Read the model definition and answer for the solid it produces. Units are mm, in the model's axes. A direction names the side the tool comes from. Coordinates: 2 decimals unless noted, no trailing zeros. Loops run counter-clockwise (first coordinate to the right, second up) from the corner with the lowest first, then second, coordinate; pieces in that order, holes last. Notation, with made-up numbers: (41.5, 18) - (80.5, 18) arc R10 cw to (80.5, 34) - close; hole circle Ø11 at (-35, 87.25). An arc over 180 degrees is marked (long way). Use CSV: the item, a comma, the result in double quotes.
Autodesk Inventor part; units mm, degrees
ref_plane "YZ Plane" through (0, 0, 0) normal (1, 0, 0) x (0, 1, 0)
ref_plane "XZ Plane" through (0, 0, 0) normal (0, 1, 0) x (-1, 0, 0)
ref_plane "XY Plane" through (0, 0, 0) normal (0, 0, 1) x (1, 0, 0)
sketch "Эскиз1" plane through (0, 0, 0) normal (0, 1, 0) x (-1, 0, 0)
  line L0 (0, 0) -> (-16, 0)
  line L1 (-16, 0) -> (-16, -7)
  line L2 (-16, -7) -> (0, -7)
  line L3 (0, -7) -> (0, 0)
  circle A0 centre (-13.5, -3.5) radius 1.5
  dimension "d0" = 16
  dimension "d1" = 7
  dimension "d2" = 3
  dimension "d3" = 2.5
  dimension "d4" = 3.5
extrude "Выдавливание1" add sketch "Эскиз1" along normal blind 5
sketch "Эскиз2" plane through (0, 0, 0) normal (0, 1, 0) x (-1, 0, 0)
  line L0 (-16, 0) -> (-16, -7) construction
  line L1 (-16, -7) -> (0, -7) construction
  line L2 (0, -7) -> (0, 0)
  line L3 (0, 0) -> (-16, 0) construction
  circle A0 centre (-13.5, -3.5) radius 1.5 construction
  line L4 (0, 0) -> (-7, 0)
  line L5 (-7, 0) -> (-7, -7)
  line L6 (-7, -7) -> (0, -7)
  line L7 (0, -7) -> (0, 0)
  point P0 (0, -7)
  dimension "d7" = 7
  dimension "d8" = 7
extrude "Выдавливание2" add sketch "Эскиз2" along normal blind 8
sketch "Эскиз3" plane through (0, 0, 0) normal (0, 0, 1) x (1, 0, 0)
  line L0 (0, 0) -> (16, 0) construction
  line L1 (16, 0) -> (16, 5) construction
  line L2 (7, 5) -> (16, 5) construction
  line L3 (7, 5) -> (7, 8) construction
  line L4 (0, 8) -> (7, 8) construction
  line L5 (0, 0) -> (0, 8) construction
  circle A0 centre (3.5, 4.5) radius 1.5
  dimension "d11" = 3
  dimension "d12" = 3.5
  dimension "d13" = 3.5
extrude "Выдавливание3" cut sketch "Эскиз3" against normal blind 7
properties part number "angle_01"
Q1. Find the intervals of material crossed by probe 1 along Z at (x, y) = (13.5, 1.8); probe 2 along X at (y, z) = (3.5, -3.75); probe 3 along Y at (x, z) = (3.5, -5.5), in increasing order. Write a range as [from, to].
Reported:
probe 1,"z = [-7, -5], [-2, 0]"
probe 2,"x = [0, 2.38], [4.62, 12.02], [14.98, 16]"
probe 3,"y = [0, 3], [6, 8]"
Q2. The part is cut by section A-A on z = -3.5. Determine the outline of the cut face in (x, y).
Reported:
outline,"(0, 0) - (12, 0) - (12, 5) - (7, 5) - (7, 8) - (0, 8) - close; (15, 0) - (16, 0) - (16, 5) - (15, 5) - close; hole circle Ø3 at (3.5, 4.5)"
Q3. The part is cut by section D-D on y = 1.75. Determine the outline of the cut face in (x, z), and give its area (3 significant figures).
Reported:
outline,"(0, -7) - (16, -7) - (16, 0) - (0, 0) - close; hole circle Ø3 at (13.5, -3.5)"
area,"105 mm²"
Q4. A tool of negligible diameter and unlimited length cuts with its end or side. For faces 1 (the face through (8, 0, -3)), 2 (the face through (11.6, 5, -3.5)), from which of +Z, -Z, +X, -X, +Y, -Y can it reach the whole face along a straight path? Write none if from no direction.
Reported:
face 1,"+Z, -Z, +X, -X, -Y"
face 2,"+Z, -Z, +X, +Y"
Q5. For a pull along Z with two mould halves and no side action, classify faces 3 (the face through (15, 2.46, -3.57)), 4 (the face through (8, 3, 0)), 5 (the face through (8, 3, -7)), 6 (the face through (16, 2, -3)) as +Z half, -Z half, draft (parallel to the pull), parting line (faces both ways), or undercut.
Reported:
face 3,"undercut"
face 4,"+Z half"
face 5,"-Z half"
face 6,"draft"
Q6. The part is cut by section C-C on x = 3.5. Determine the outline of the cut face in (y, z).
Reported:
outline,"(0, -7) - (3, -7) - (3, 0) - (0, 0) - close; (6, -7) - (8, -7) - (8, 0) - (6, 0) - close"
Q7. The part is cut by section B-B on y = 4.5. Determine the outline of the cut face in (x, z).
Reported:
outline,"(0, -7) - (2, -7) - (2, 0) - (0, 0) - close; (5, -7) - (16, -7) - (16, 0) - (5, 0) - close; hole circle Ø3 at (13.5, -3.5)"
Q8. Given P1, Ø0.9, axis at y = 6.5, z = -2, coming from the +X side, flat-ended and moving along its own axis, determine where the tip first touches the part or whether it passes through.
Reported:
P1,"stops at x = 7"
